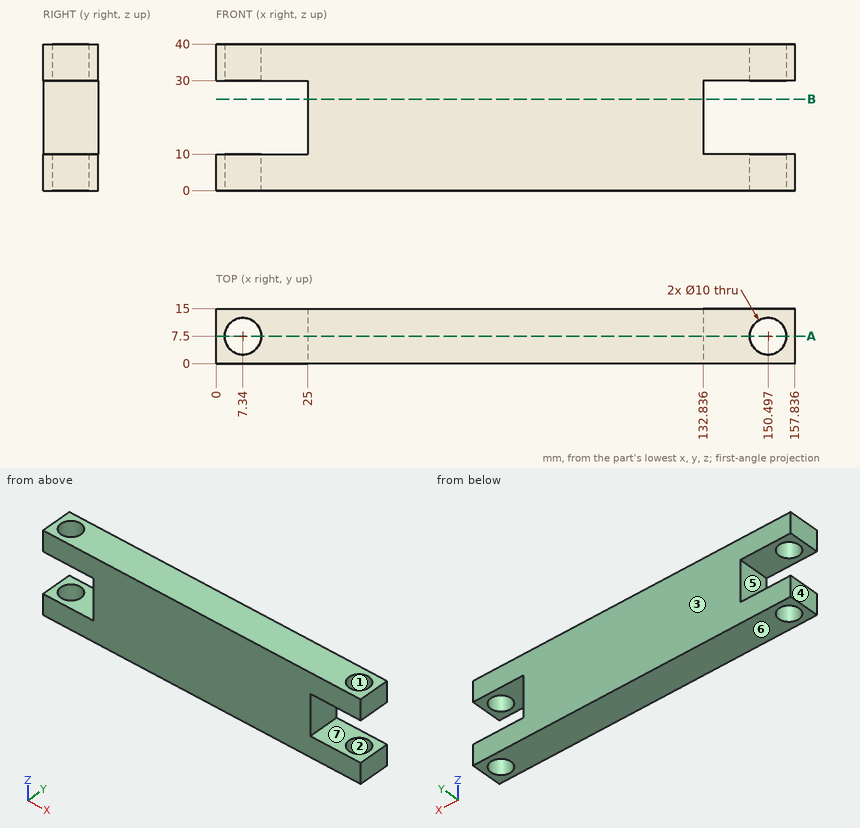
Verification items for this drawing (mm, ordinates from the low corner). A direction names the side the tool comes from. Give positions to 0.01 mm unless a question says otherwise; leave off trailing zeros. Order: outer loops, then holes, each group sorted by start corner. A loop starts at its lowest first (then second) coordinate and runs counter-clockwise, first axis right, second up. Notation, with made-up numbers: M 56.5,-12 L 101.5,-12 A23 ccw 101.5,12 Z; hole C 37.5,-23 d10. An arc over 180 degrees is marked long. Use a Markdown table: item, result.
Item 1: Section check B-B (z = 25). Record the cut outline in (x, y).
Answers follow:
| item | result |
|---|---|
| outline | M 25,0 L 132.84,0 L 132.84,15 L 25,15 Z |
Item 2: Section check A-A (y = 7.5). Record the cut outline in (x, z), and give its area (3 significant figures).
Answers follow:
| item | result |
|---|---|
| outline | M 0,0 L 2.34,0 L 2.34,10 L 0,10 Z; M 0,30 L 2.34,30 L 2.34,40 L 0,40 Z; M 12.34,0 L 145.5,0 L 145.5,10 L 132.84,10 L 132.84,30 L 145.5,30 L 145.5,40 L 12.34,40 L 12.34,30 L 25,30 L 25,10 L 12.34,10 Z; M 155.5,0 L 157.84,0 L 157.84,10 L 155.5,10 Z; M 155.5,30 L 157.84,30 L 157.84,40 L 155.5,40 Z |
| area | 4,910 mm2 |
Item 3: Tool access check on the marked faces 5, 6 and 7. Record the directions out of +Z, -Z, +X, -X, +Y, -Y that give a thin tool (end or side, any length) a straight path to the whole face; none if there is none.
Answers follow:
| item | result |
|---|---|
| face 5 | -X, +Y, -Y |
| face 6 | -Z, +X, -X, +Y, -Y |
| face 7 | +X, +Y, -Y |
Item 4: Depth check by flat-ended pin: P1, Ø1.5, axis at y = 10, z = 17.5, coming from the -X side; P2, Ø3, axis at y = 5, z = 26, coming from the +X side; P3, Ø9, axis at x = 150.5, y = 7.5, coming from the +Z side. Enter the tip coordinate at first touch or a pass-through.
Answers follow:
| item | result |
|---|---|
| P1 | stops at x = 25 |
| P2 | stops at x = 132.84 |
| P3 | passes through |
Item 5: Material ranges on line 1 along X through (y, z) = (7.5, 36.25); line 2 along Z through (x, y) = (145.5, 10.75); line 3 along X through (y, z) = (9, 36), recorded low to high.
Answers follow:
| item | result |
|---|---|
| line 1 | x = 0 to 2.34, 12.34 to 145.5, 155.5 to 157.84 |
| line 2 | z = 0 to 10, 30 to 40 |
| line 3 | x = 0 to 2.57, 12.11 to 145.73, 155.27 to 157.84 |
Item 6: Draft check along X on the marked faces 1, 2, 3 and 4. Enter one of: +X half, -X half, draft (parallel to the pull), parting line (faces both ways), or undercut.
Answers follow:
| item | result |
|---|---|
| face 1 | undercut |
| face 2 | undercut |
| face 3 | draft |
| face 4 | -X half |
